from build123d import *

# Parameters (mm, degrees)
CHAMFER_1_SIZE = 3


with BuildPart() as part:
    # Эскиз1 → Повернуть1 (revolve)
    with BuildSketch(Plane.XY):
        with BuildLine():
            Line((6, 18), (6, 23.5))
            Line((6, 23.5), (-8, 23.5))
            Line((-8, 23.5), (-8, 25.5))
            Line((-8, 25.5), (-9.7, 25.5))
            Line((-9.7, 25.5), (-9.7, 23.5))
            Line((-9.7, 23.5), (-19, 23.5))
            Line((-19, 23.5), (-19, 29.75))
            Line((-19, 29.75), (-10, 29.75))
            Line((-10, 29.75), (-10, 38.5))
            Line((-10, 38.5), (-6, 63.5))
            ThreePointArc((-6, 63.5), (0, 64.5), (6, 63.5))
            Line((6, 63.5), (10, 38.5))
            Line((10, 38.5), (10, 18))
            ThreePointArc((10, 18), (14.460498942, 9.486832981), (16, 0))
            Line((16, 0), (12.907248094, 0))
            ThreePointArc((12.907248094, 0), (11.121156043, 9.639892067), (6, 18))
        make_face()
    revolve(axis=Axis((12.907248094, 0, 0), (1, 0, 0)))

    # Фаска1
    chamfer_1_edges = [part.edges().sort_by_distance(p)[0] for p in [
        (-19, -29.75, 0),
    ]]
    chamfer(chamfer_1_edges, length=CHAMFER_1_SIZE)


solid = part.part
Can you work these out from the model? Positions are in its coordinate system, mm. A direction names the side the tool comes from. Give positions to 0.01 mm unless a question says otherwise; leave off trailing zeros. Write each loop counter-clockwise with the first axis right and the second up, starting at its lowest first coordinate (ties: lowest second). Pieces come first, ordered by that corner, then holes. Notation, with made-up numbers: M 78,35 L 111,35 A18 ccw 111,39 Z; hole C 11,17.5 d9. An arc over 180 degrees is marked long. Answer in a Markdown table with one row per item. Add a question column.
Item 1: Please list where these lines run through material, in increasing order: L1, parallel to X at y = -24, z = -4; L2, parallel to Z at x = -1, y = 0; L3, parallel to Y at x = -1, z = 8.
Item 2: Imagine slicing it at C-C, the plane x = -12.5. Write out the boundary of the cut face in (y, z).
Item 3: We'd pull the mould along X, two halves only. Please class faces 4 (the cylindrical face through (-14.4, 22.4, 7.1)), 5 (the flat face through (-8, -11, -21)), 6 (the flat face through (10, 8, -17)): released by +X, released by -X, zero draft, split by the parting line, or undercut.
Item 4: On a 3-axis mill with a long thin cutter (end or side, diameter ignored), from which of +Z, -Z, +X, -X, +Y, -Y can I reach the whole of each face in a straight line? I mean faces 1 (the flat face through (-9.7, 11, -21)), 2 (the flat face through (-19, 0, -24)), 3 (the flat face through (-10, -20, -23)). Say none if no direction works.
Item 5: For pin 1 Ø1 at (x, y) = (-5, 38) entering from -Z; pin 2 Ø1.5 at (x, y) = (-2.5, -31) entering from -Z; pin 3 Ø12 at (x, z) = (8, -29.5) entering from -Y, each with a flat end and sliding along its axis, tell me the tip position at first contact or that it passes through.
Item 6: Imagine slicing it at D-D, the plane x = 3.5. Write out the boundary of the cut face in (y, z), plus the area to 3 significant figures.
Evaluation:
| question | item | result |
|---|---|---|
| 1 | L1 | x = -19 to -9.7, -8 to 10 |
| 1 | L2 | z = -64.47 to -23.5, 23.5 to 64.47 |
| 1 | L3 | y = -63.97 to -22.1, 22.1 to 63.97 |
| 2 | outline | C 0,0 d59.5; hole C 0,0 d47 |
| 3 | face 4 | zero draft |
| 3 | face 5 | undercut |
| 3 | face 6 | released by +X |
| 4 | face 1 | none |
| 4 | face 2 | +Z, -Z, -X, +Y, -Y |
| 4 | face 3 | -X |
| 5 | pin 1 | stops at z = -51.67 |
| 5 | pin 2 | stops at z = -56.79 |
| 5 | pin 3 | stops at y = -59.01 |
| 6 | outline | C 0,0 d128.33; hole C 0,0 d47 |
| 6 | area | 11,200 mm² |
